Check sheet for the drawn part. Datum: minimum x, y, z corner. Units: mm. A direction names the side the tool comes from. Coordinates: 2 decimals unless noted, no trailing zeros. Write each loop counter-clockwise with the first axis right and the second up, starting at its lowest first coordinate (ties: lowest second). Pieces come first, ordered by that corner, then holes. Notation, with made-up numbers: (38, 82) -> (84, 82) arc R20 cw to (84, 93) -> close; hole circle Ø11 at (-20, -6). An arc over 180 degrees is marked (long way). Answer in a Markdown table with one row per item.
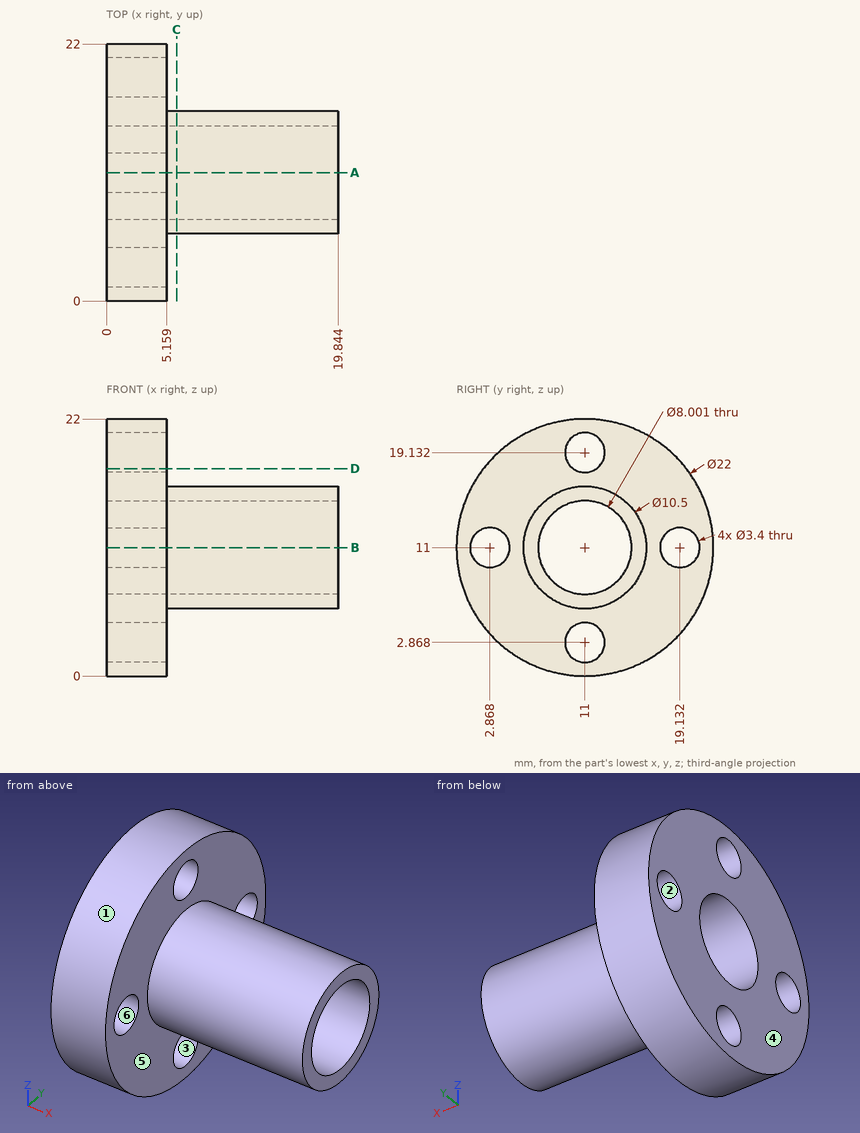
1. Release check for a two-part mould opening along Z. For the marked faces 1, 2, 3 and 4 record: released by +Z, released by -Z, zero draft, split by the parting line, or undercut.
Findings below:
| item | result |
|---|---|
| face 1 | split by the parting line |
| face 2 | undercut |
| face 3 | undercut |
| face 4 | zero draft |
2. Go/stop test with flat-tipped pins: pin 1 (3 mm diameter, centred on x = 7, y = 6, fed in from -Z); pin 2 (13 mm diameter, centred on y = 11, z = 11, fed in from +X); pin 3 (8 mm diameter, centred on x = 4, y = 2.5, fed in from -Z); pin 4 (2 mm diameter, centred on x = 12, z = 10, fed in from -Y). Record where each tip stops, or that it passes through.
Findings below:
| item | result |
|---|---|
| pin 1 | stops at z = 7.09 |
| pin 2 | stops at x = 19.84 |
| pin 3 | stops at z = 0.96 |
| pin 4 | stops at y = 5.75 |
3. Material ranges on probe 1 along Y at (x, z) = (4.5, 11); probe 2 along Z at (x, y) = (6.75, 11.25) (1 decimal); probe 3 along Y at (x, z) = (6.5, 11), recorded low to high. Write a range as from..to.
Findings below:
| item | result |
|---|---|
| probe 1 | y = 0..1.17, 4.57..7, 15..17.43, 20.83..22 |
| probe 2 | z = 5.8..7, 15..16.2 |
| probe 3 | y = 5.75..7, 15..16.25 |
4. Sectioned sample at D-D, the plane z = 17.75. Record the cut outline in (x, y) (1 decimal).
Findings below:
| item | result |
|---|---|
| outline | (0, 2.3) -> (5.2, 2.3) -> (5.2, 10) -> (0, 10) -> close; (0, 12) -> (5.2, 12) -> (5.2, 19.7) -> (0, 19.7) -> close |
5. Sectioned sample at A-A, the plane y = 11. Record the cut outline in (x, z).
Findings below:
| item | result |
|---|---|
| outline | (0, 0) -> (5.16, 0) -> (5.16, 1.17) -> (0, 1.17) -> close; (0, 4.57) -> (5.16, 4.57) -> (5.16, 5.75) -> (19.84, 5.75) -> (19.84, 7) -> (0, 7) -> close; (0, 15) -> (19.84, 15) -> (19.84, 16.25) -> (5.16, 16.25) -> (5.16, 17.43) -> (0, 17.43) -> close; (0, 20.83) -> (5.16, 20.83) -> (5.16, 22) -> (0, 22) -> close |
6. Sectioned sample at C-C, the plane x = 6. Record the cut outline in (y, z).
Findings below:
| item | result |
|---|---|
| outline | circle Ø10.5 at (11, 11); hole circle Ø8 at (11, 11) |
7. Access from +Z, -Z, +X, -X, +Y, -Y to the whole of each face (thin tool, end or side, straight path). Record for the marked faces 5 and 6.
Findings below:
| item | result |
|---|---|
| face 5 | +X |
| face 6 | +X, -X |
